```python
from build123d import *

# Parameters (mm, degrees)
ESQUISSE1_W             = 150
ESQUISSE1_H             = 240
BOSS_EXTRU_1_DEPTH      = 50
ESQUISSE2_W             = 140
ESQUISSE2_H             = 230
ENL_V_MAT_EXTRU_1_DEPTH = 46
ESQUISSE3_W             = 101.7
ESQUISSE3_H             = 167
ENL_V_MAT_EXTRU_2_DEPTH = 151.083310198
CONG_1_R                = 5


with BuildPart() as part:
    # Esquisse1 → Boss.-Extru.1 (new body)
    with BuildSketch(Plane.XY):
        Rectangle(ESQUISSE1_W, ESQUISSE1_H)
    extrude(amount=BOSS_EXTRU_1_DEPTH)

    # Esquisse2 → Enlèv. mat.-Extru.1 (cut)
    with BuildSketch(Plane(origin=(0, 0, 0), x_dir=(-1, 0, 0), z_dir=(0, 0, -1))):
        Rectangle(ESQUISSE2_W, ESQUISSE2_H)
    extrude(amount=-ENL_V_MAT_EXTRU_1_DEPTH, mode=Mode.SUBTRACT)

    # Esquisse3 → Enlèv. mat.-Extru.2 (cut, through all)
    with BuildSketch(Plane.XY.offset(50)):
        with Locations((0, 26.5)):
            Rectangle(ESQUISSE3_W, ESQUISSE3_H)
    extrude(amount=-ENL_V_MAT_EXTRU_2_DEPTH, mode=Mode.SUBTRACT)

    # Congé1
    cong_1_edges = [part.edges().sort_by_distance(p)[0] for p in [
        (-75, 120, 25),
        (75, 120, 25),
        (75, -120, 25),
        (-75, -120, 25),
    ]]
    fillet(cong_1_edges, radius=CONG_1_R)


solid = part.part
```
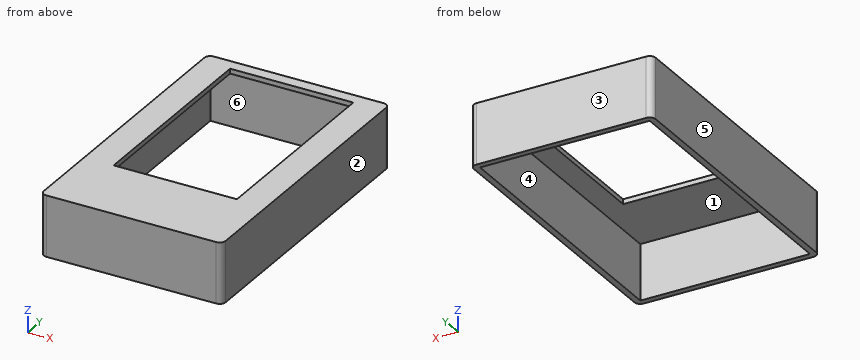
Could you check a few things on this model? Use its own coordinates, in mm. Face numbers are marked on the shaded views. A direction names the side the tool comes from. Round coordinates to 2 decimals unless told otherwise and drop trailing zeros. Write each loop counter-clockwise with the first axis right and the second up, starting at its lowest first coordinate (ties: lowest second). Pieces come first, ordered by that corner, then holes. Notation, with made-up numbers: M 55,19 L 106,19 A8 ccw 106,32 Z; hole C 54,49.25 d6. An arc over 180 degrees is marked long. Answer in a Markdown table with one row per item. Add a question column.
Q1. Imagine slicing it at A-A (y = -49). Please give me the cut outline in (x, z), then the cut area to 3 significant figures.
Q2. Imagine slicing it at D-D (y = -99). Please give me the cut outline in (x, z), then the cut area to 3 significant figures.
Q3. On a 3-axis mill with a long thin cutter (end or side, diameter ignored), from which of +Z, -Z, +X, -X, +Y, -Y can I reach the whole of each face in a straight line? I mean the marked faces 1 and 2. Say none if no direction works.
Q4. If I drill on line 1 (Y direction, x = 28, z = 5.5); line 2 (X direction, y = 27, z = 7.5); line 3 (Y direction, x = 46, z = 47), over which ranges is the centre line in solid material (lowest first)? Write a range as from..to.
Q5. If we mould it in two halves opening along X, with no side actions, what happens to the marked faces 3, 4, 5 and 6? For each: +X half, -X half, draft (parallel to the pull), parting line (faces both ways), or undercut.
Q6. Imagine slicing it at B-B (z = 27). Please give me the cut outline in (x, y), then the cut area to 3 significant figures.
Q7. Imagine slicing it at C-C (x = -5.5). Please give me the cut outline in (y, z), then the cut area to 3 significant figures.
Values:
| question | item | result |
|---|---|---|
| 1 | outline | M -75,0 L -70,0 L -70,46 L -50.85,46 L -50.85,50 L -75,50 Z; M 50.85,46 L 70,46 L 70,0 L 75,0 L 75,50 L 50.85,50 Z |
| 1 | area | 653 mm^2 |
| 2 | outline | M -75,0 L -70,0 L -70,46 L 70,46 L 70,0 L 75,0 L 75,50 L -75,50 Z |
| 2 | area | 1,060 mm^2 |
| 3 | face 1 | -Z |
| 3 | face 2 | +Z, -Z, +X, +Y, -Y |
| 4 | line 1 | -120..-115, 115..120 |
| 4 | line 2 | -75..-70, 70..75 |
| 4 | line 3 | -120..-57, 110..120 |
| 5 | face 3 | draft |
| 5 | face 4 | undercut |
| 5 | face 5 | -X half |
| 5 | face 6 | undercut |
| 6 | outline | M -75,-115 A5 ccw -70,-120 L 70,-120 A5 ccw 75,-115 L 75,115 A5 ccw 70,120 L -70,120 A5 ccw -75,115 Z; hole M -70,-115 L 70,-115 L 70,115 L -70,115 Z |
| 6 | area | 3,780 mm^2 |
| 7 | outline | M -120,0 L -115,0 L -115,46 L -57,46 L -57,50 L -120,50 Z; M 110,46 L 115,46 L 115,0 L 120,0 L 120,50 L 110,50 Z |
| 7 | area | 752 mm^2 |
